```python
from build123d import *

# Parameters (mm, degrees)
MODEL_W                 = 3
MODEL_H                 = 3
SALIENTE_EXTRUIR1_DEPTH = 3


with BuildPart() as part:
    # Model → Saliente-Extruir1 (new body)
    with BuildSketch(Plane.XY):
        with BuildLine():
            Line((36.621026826, 298.155466529), (39.023886305, 298.155466529))
            ThreePointArc((39.023886305, 298.155466529), (40.044302886, 297.82717325), (40.681867004, 296.965466529))
            ThreePointArc((40.681867004, 296.965466529), (40.614360153, 296.513918935), (40.208158233, 296.305466529))
            Line((40.208158233, 296.305466529), (39.721026826, 296.305466529))
            Line((39.721026826, 296.305466529), (39.721026826, 293.405466529))
            Line((39.721026826, 293.405466529), (41.121026826, 293.405466529))
            Line((41.121026826, 293.405466529), (41.121026826, 266.405466529))
            Line((41.121026826, 266.405466529), (39.721026826, 266.405466529))
            Line((39.721026826, 266.405466529), (39.721026826, 263.505466529))
            Line((39.721026826, 263.505466529), (40.208158233, 263.505466529))
            ThreePointArc((40.208158233, 263.505466529), (40.614360153, 263.297014124), (40.681867004, 262.845466529))
            ThreePointArc((40.681867004, 262.845466529), (40.044302886, 261.983759808), (39.023886305, 261.655466529))
            Line((39.023886305, 261.655466529), (36.621026826, 261.655466529))
            Line((36.621026826, 261.655466529), (36.621026826, 273.405466529))
            ThreePointArc((36.621026826, 273.405466529), (36.401356911, 273.935796615), (35.871026826, 274.155466529))
            Line((35.871026826, 274.155466529), (34.371026826, 274.155466529))
            ThreePointArc((34.371026826, 274.155466529), (33.84069674, 273.935796615), (33.621026826, 273.405466529))
            Line((33.621026826, 273.405466529), (33.621026826, 266.405466529))
            Line((33.621026826, 266.405466529), (18.621026826, 266.405466529))
            Line((18.621026826, 266.405466529), (18.621026826, 273.405466529))
            ThreePointArc((18.621026826, 273.405466529), (18.401356911, 273.935796615), (17.871026826, 274.155466529))
            Line((17.871026826, 274.155466529), (16.371026826, 274.155466529))
            ThreePointArc((16.371026826, 274.155466529), (15.84069674, 273.935796615), (15.621026826, 273.405466529))
            Line((15.621026826, 273.405466529), (15.621026826, 261.655466529))
            Line((15.621026826, 261.655466529), (13.218167347, 261.655466529))
            ThreePointArc((13.218167347, 261.655466529), (12.197750765, 261.983759808), (11.560186647, 262.845466529))
            ThreePointArc((11.560186647, 262.845466529), (11.627693498, 263.297014124), (12.033895418, 263.505466529))
            Line((12.033895418, 263.505466529), (12.521026826, 263.505466529))
            Line((12.521026826, 263.505466529), (12.521026826, 266.405466529))
            Line((12.521026826, 266.405466529), (11.121026826, 266.405466529))
            Line((11.121026826, 266.405466529), (11.121026826, 293.405466529))
            Line((11.121026826, 293.405466529), (12.521026826, 293.405466529))
            Line((12.521026826, 293.405466529), (12.521026826, 296.305466529))
            Line((12.521026826, 296.305466529), (12.033895418, 296.305466529))
            ThreePointArc((12.033895418, 296.305466529), (11.627693498, 296.513918935), (11.560186647, 296.965466529))
            ThreePointArc((11.560186647, 296.965466529), (12.197750765, 297.82717325), (13.218167347, 298.155466529))
            Line((13.218167347, 298.155466529), (15.621026826, 298.155466529))
            Line((15.621026826, 298.155466529), (15.621026826, 286.405466529))
            ThreePointArc((15.621026826, 286.405466529), (15.84069674, 285.875136443), (16.371026826, 285.655466529))
            Line((16.371026826, 285.655466529), (17.871026826, 285.655466529))
            ThreePointArc((17.871026826, 285.655466529), (18.401356911, 285.875136443), (18.621026826, 286.405466529))
            Line((18.621026826, 286.405466529), (18.621026826, 293.405466529))
            Line((18.621026826, 293.405466529), (33.621026826, 293.405466529))
            Line((33.621026826, 293.405466529), (33.621026826, 286.405466529))
            ThreePointArc((33.621026826, 286.405466529), (33.84069674, 285.875136443), (34.371026826, 285.655466529))
            Line((34.371026826, 285.655466529), (35.871026826, 285.655466529))
            ThreePointArc((35.871026826, 285.655466529), (36.401356911, 285.875136443), (36.621026826, 286.405466529))
            Line((36.621026826, 286.405466529), (36.621026826, 298.155466529))
        make_face()
        with Locations((26.121026826, 288.905466529)):
            Rectangle(MODEL_W, MODEL_H, mode=Mode.SUBTRACT)
        with Locations((17.121026826, 279.905466529)):
            Rectangle(MODEL_W, MODEL_H, mode=Mode.SUBTRACT)
        with Locations((26.121026826, 279.905466529)):
            Rectangle(MODEL_W, MODEL_H, mode=Mode.SUBTRACT)
        with Locations((26.121026826, 270.905466529)):
            Rectangle(MODEL_W, MODEL_H, mode=Mode.SUBTRACT)
        with Locations((35.121026826, 279.905466529)):
            Rectangle(MODEL_W, MODEL_H, mode=Mode.SUBTRACT)
    extrude(amount=SALIENTE_EXTRUIR1_DEPTH)


solid = part.part
```
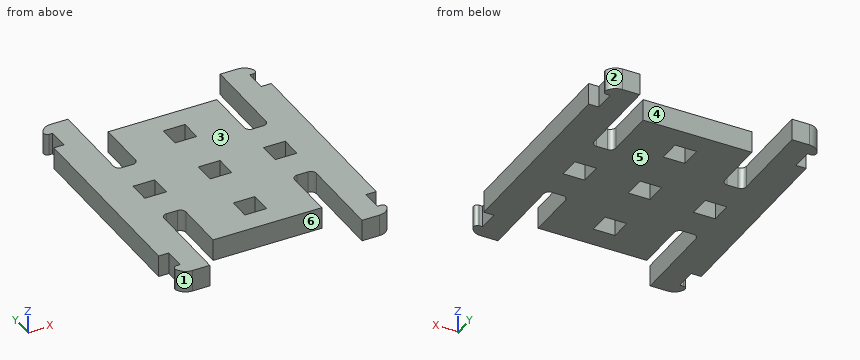
The model under review builds one solid part; all positions refer to its coordinate system, in mm. Face numbers are marked on the shaded views. A direction names the side the tool comes from. Give positions to 0.01 mm unless a question says otherwise; leave off trailing zeros. Write each loop counter-clockwise with the first axis right and the second up, starting at its lowest first coordinate (ties: lowest second). Pieces come first, ordered by that corner, then holes.
(1) Tool access review of the marked faces 5 and 6: name each direction out of +Z, -Z, +X, -X, +Y, -Y from which nothing blocks a thin tool from reaching the whole face with its end or side.
(2) To check wall thickness, follow L1, parallel to X at y = 289, z = 0.7; L2, parallel to X at y = 269, z = 1.4; L3, parallel to Y at x = 25.5, z = 1.3. State the ranges of each line that lie inside material, in increasing order.
(3) Consider section B-B, the plane y = 269. Give the boundary of the cut face in (x, z), and give its area (3 significant figures).
(4) Consider section A-A, the plane x = 25.25. Give the boundary of the cut face in (y, z), and give its area (3 significant figures).
(5) Consider section D-D, the plane x = 29.5. Give the boundary of the cut face in (y, z).
(6) Consider section C-C, the plane z = 0.65. Give the number of separate pieces and of enclosed holes in the cut face, and give its area (3 significant figures).
(7) For P1, Ø1.2, axis at x = 17.5, z = 1.5, coming from the -Y side; P2, Ø0.9, axis at x = 35.5, z = 2, coming from the -Y side; P3, Ø5, axis at x = 37.5, y = 269.5, coming from the -Z side; P4, Ø1.5, axis at x = 25.5, z = 1.5, coming from the -Y side, all flat-tipped, find the tip position at first contact; note any pin that passes through.
(8) The part is to be moulded in two halves that separate along X. For the marked faces 1, 2, 3 and 4, say which applies: released by +X, released by -X, zero draft, split by the parting line, or undercut.
Returned:
1. face 5: -Z, +X, -X, +Y, -Y
1. face 6: +Z, -Z, -Y
2. L1: x = 11.12 to 15.62, 18.62 to 24.62, 27.62 to 33.62, 36.62 to 41.12
2. L2: x = 11.12 to 15.62, 18.62 to 33.62, 36.62 to 41.12
2. L3: y = 266.41 to 269.41, 272.41 to 278.41, 281.41 to 287.41, 290.41 to 293.41
3. outline: (11.12, 0) - (15.62, 0) - (15.62, 3) - (11.12, 3) - close; (18.62, 0) - (33.62, 0) - (33.62, 3) - (18.62, 3) - close; (36.62, 0) - (41.12, 0) - (41.12, 3) - (36.62, 3) - close
3. area: 72.0 mm2
4. outline: (266.41, 0) - (269.41, 0) - (269.41, 3) - (266.41, 3) - close; (272.41, 0) - (278.41, 0) - (278.41, 3) - (272.41, 3) - close; (281.41, 0) - (287.41, 0) - (287.41, 3) - (281.41, 3) - close; (290.41, 0) - (293.41, 0) - (293.41, 3) - (290.41, 3) - close
4. area: 54.0 mm2
5. outline: (266.41, 0) - (293.41, 0) - (293.41, 3) - (266.41, 3) - close
6. separate pieces: 1
6. enclosed holes: 5
6. area: 737 mm2
7. P1: stops at y = 274.12
7. P2: stops at y = 274.15
7. P3: stops at z = 0
7. P4: stops at y = 266.41
8. face 1: released by -X
8. face 2: released by +X
8. face 3: zero draft
8. face 4: undercut
